Geometry check sheet. Reference: the model listing, model coordinates, mm. A direction names the side the tool comes from. Round coordinates to 2 decimals unless told otherwise and drop trailing zeros. Write each loop counter-clockwise with the first axis right and the second up, starting at its lowest first coordinate (ties: lowest second). Pieces come first, ordered by that corner, then holes. Notation, with made-up numbers: (52.25, -20) - (98.25, -20) arc R23 cw to (98.25, -6) - close; hole circle Ø10 at (86, -5.5). An arc over 180 degrees is marked (long way). Return JSON: item names as keys, results as strings.
```python
from build123d import *

# Parameters (mm, degrees)
SKIZZE1_R                       = 25
AUFSATZ_LINEAR_AUSTRAGEN1_DEPTH = 200
SCHNITT_LINEAR_AUSTRAGEN1_DEPTH = 10


with BuildPart() as part:
    # Skizze1 → Aufsatz-Linear austragen1 (new body)
    with BuildSketch(Plane(origin=(0, 0, 0), x_dir=(1, 0, 0), z_dir=(0, 1, 0))):
        with Locations(Location((0, 0, 0), (0, 0, 270))):  # turned: the seam where the file's is
            Circle(SKIZZE1_R)
    extrude(amount=AUFSATZ_LINEAR_AUSTRAGEN1_DEPTH)

    # Skizze2 → Schnitt-Linear austragen1 (cut)
    with BuildSketch(Plane.XY.offset(25)):
        with BuildLine():
            Line((-4.234822954, 21.641230775), (-4.234822954, 34.628021169))
            ThreePointArc((-4.234822954, 34.628021169), (0, 38.862844123), (4.234822954, 34.628021169))
            Line((4.234822954, 34.628021169), (4.234822954, 21.641230775))
            ThreePointArc((4.234822954, 21.641230775), (0, 17.406407821), (-4.234822954, 21.641230775))
        make_face()
    extrude(amount=-SCHNITT_LINEAR_AUSTRAGEN1_DEPTH, mode=Mode.SUBTRACT)


solid = part.part
```
(1) Section check C-C, the plane z = -6.5. Enter the section's corners in (x, y).
Response values:
{"outline": "(-24.14, 0) - (24.14, 0) - (24.14, 200) - (-24.14, 200) - close"}
(2) Access from +Z, -Z, +X, -X, +Y, -Y to the whole of each face (thin tool, end or side, straight path). Record for faces 1 (the face through (7.509, 98.6, 23.846)), 2 (the face through (0, 28, 15)).
Response values:
{"face 1": "+Y, -Y", "face 2": "+Z"}
(3) Section check A-A, the plane x = 0. Enter the section's corners in (y, z).
Response values:
{"outline": "(0, -25) - (200, -25) - (200, 25) - (38.86, 25) - (38.86, 15) - (17.41, 15) - (17.41, 25) - (0, 25) - close"}
(4) Gauge pin test, flat ends, axial feed: pin 1 (3 mm diameter, centred on y = 131, z = -18.5, fed in from -X); pin 2 (8 mm diameter, centred on y = 27, z = -5.5, fed in from +X); pin 3 (5 mm diameter, centred on y = 28, z = 21, fed in from -X). Record the tip position at first contact, or that the pin passes through.
Response values:
{"pin 1": "stops at x = -18.33", "pin 2": "stops at x = 24.95", "pin 3": "stops at x = -16.82"}
(5) Section check D-D, the plane z = -21. Enter the section's corners in (x, y).
Response values:
{"outline": "(-13.56, 0) - (13.56, 0) - (13.56, 200) - (-13.56, 200) - close"}
(6) Material ranges on line 1 along X through (y, z) = (115, -2); line 2 along Z through (x, y) = (-7.5, 42); line 3 along Z through (x, y) = (12, 179), recorded low to high. Write a range as [from, to].
Response values:
{"line 1": "x = [-24.92, 24.92]", "line 2": "z = [-23.85, 23.85]", "line 3": "z = [-21.93, 21.93]"}
(7) Release check for a two-part mould opening along Y. For faces 3 (the face through (0, 0, 0)), 4 (the face through (0, 200, 0)), 5 (the face through (4.235, 28, 20)) record: pulls with the +Y half, pulls with the -Y half, needs draft (parallel to the pull), parting line crosses it, or undercut.
Response values:
{"face 3": "pulls with the -Y half", "face 4": "pulls with the +Y half", "face 5": "undercut"}
(8) Section check B-B, the plane y = 127.5. Enter the section's corners in (x, z), plus the area to 3 significant figures.
Response values:
{"outline": "circle Ø50 at (0, 0)", "area": "1,960 mm^2"}
